Part model, mm, in its own coordinate system. A direction names the side the tool comes from. Give positions to 0.01 mm unless a question says otherwise; leave off trailing zeros. Write each loop counter-clockwise with the first axis right and the second up, starting at its lowest first coordinate (ties: lowest second). Pieces come first, ordered by that corner, then holes. Notation, with made-up numbers: (-23.75, 33) - (-10.75, 33) arc R9 cw to (-10.75, 48) - close; hole circle Ø2 at (47, 36). An arc over 180 degrees is marked (long way). Answer in a Markdown table with one row per item. Add a question column.
1. Band-saw the part on A-A on y = 8. State how many separate pieces and enclosed holes the cut face has, plus the area to 3 significant figures.
2. Pull direction Z, two halves, no side cores. Call faces 5 (the cylindrical face through (-5.08, -0.07, -25.92)), 6 (the cylindrical face through (-24.89, -0.07, 8.62)), 7 (the flat face through (24.3, 41, -39)): released by +Z, released by -Z, zero draft, split by the parting line, or undercut.
3. Band-saw the part on C-C on x = -4. Write the cut outline in (y, z).
4. Drop flat-ended pins along their axis: pin 1 Ø10 at (x, y) = (30.5, 23.5) entering from +Z; pin 2 Ø5 at (x, y) = (-39.5, -1) entering from +Z; pin 3 Ø1.5 at (x, z) = (-24, -2.5) entering from +Y. Give the stop position or say it passes through.
5. Probe line 1 along Z through (x, y) = (-23.75, 27.5); line 2 along Z through (x, y) = (0, 1); line 3 along Y through (x, z) = (-15, 32). List the from-to ranges inside material, lowest first.
6. Band-saw the part on B-B on z = 5. Write the cut outline in (x, y), plus the area to 3 significant figures.
7. Band-saw the part on D-D on x = -42. Write the cut outline in (y, z), plus the area to 3 significant figures.
8. Which spindle directions (+Z, -Z, +X, -X, +Y, -Y) get a long thin tool onto all of the face, cutting with end or side? Do faces 1 (the flat face through (12.522, 0.07, -36.689)), 2 (the cylindrical face through (24.89, -0.07, -8.62)), 3 (the cylindrical face through (-24.99, -0.07, -8.56)), 4 (the flat face through (-12.522, 0.07, 36.689)). Say none if no direction does.
```python
from build123d import *
from build123d.topology import SkipClean

# Parameters (mm, degrees)
SKETCH1_R                  = 25
SKETCH1_R_2                = 15
BOSS_EXTRUDE1_DEPTH        = 5
BOSS_EXTRUDE2_START        = -10
BOSS_EXTRUDE2_DEPTH        = 10
BOSS_EXTRUDE4_START        = 36
SKETCH8_R                  = 7.5
BOSS_EXTRUDE4_DEPTH        = 36
TAP_DRILL_FOR_10_32_TAP1_D = 4.0386
CIRPATTERN2_COUNT          = 6
FILLET1_R                  = 7.5


with BuildPart() as part:
    # Sketch1 → Boss-Extrude1 (new, symmetric)
    with BuildSketch(Plane(origin=(0, 0, 0), x_dir=(1, 0, 0), z_dir=(0, 1, 0))):
        with Locations(Location((0, 0, 0), (0, 0, 270))):
            Circle(SKETCH1_R)
        with Locations(Location((0, 0, 0), (0, 0, 270))):
            Circle(SKETCH1_R_2, mode=Mode.SUBTRACT)
    boss_extrude1 = extrude(amount=BOSS_EXTRUDE1_DEPTH, both=True)

    # Sketch2 → Boss-Extrude2 (add)
    with BuildSketch(Plane.XZ.offset(5).offset(BOSS_EXTRUDE2_START)):
        with BuildLine():
            ThreePointArc((55, 0), (52.803300859, 5.303300859), (47.5, 7.5))
            Line((47.5, 7.5), (23.848480035, 7.5))
            ThreePointArc((23.848480035, 7.5), (24.710443145, 3.793942482), (25, 0))
            ThreePointArc((25, 0), (24.710443145, -3.793942482), (23.848480035, -7.5))
            Line((23.848480035, -7.5), (47.5, -7.5))
            ThreePointArc((47.5, -7.5), (52.803300859, -5.303300859), (55, 0))
        make_face()
    boss_extrude2 = extrude(amount=BOSS_EXTRUDE2_DEPTH)

    # Sketch8 → Boss-Extrude4 (add)
    with SkipClean():  # the faces are left unmerged after this step: merging them gives an invalid solid
        with BuildSketch(Plane(origin=(0, 5, 0), x_dir=(1, 0, 0), z_dir=(0, 1, 0)).offset(BOSS_EXTRUDE4_START)):
            with Locations(Location((47.5, 0, 0), (0, 0, 270))):
                Circle(SKETCH8_R)
        boss_extrude4 = extrude(amount=-BOSS_EXTRUDE4_DEPTH)

    # Tap Drill for #10-32 Tap1 (through all)
    with Locations(Plane(origin=(0, -5, 0), x_dir=(-1, 0, 0), z_dir=(0, -1, 0))):
        with Locations((-47.5, 0)):
            tap_drill_for_10_32_tap1 = Hole(TAP_DRILL_FOR_10_32_TAP1_D / 2)

    # CirPattern2: Boss-Extrude1, Boss-Extrude2, Boss-Extrude4, Tap Drill for #10-32 Tap1 ×6 about axis
    cirpattern2_axis = Axis((0, 0, 0), (0, 1, 0))
    add([boss_extrude1.rotate(cirpattern2_axis, i * 360 / CIRPATTERN2_COUNT) for i in range(1, CIRPATTERN2_COUNT)])
    add([boss_extrude2.rotate(cirpattern2_axis, i * 360 / CIRPATTERN2_COUNT) for i in range(1, CIRPATTERN2_COUNT)])
    add([boss_extrude4.rotate(cirpattern2_axis, i * 360 / CIRPATTERN2_COUNT) for i in range(1, CIRPATTERN2_COUNT)])
    add([tap_drill_for_10_32_tap1.rotate(cirpattern2_axis, i * 360 / CIRPATTERN2_COUNT) for i in range(1, CIRPATTERN2_COUNT)], mode=Mode.SUBTRACT)

    # Fillet1
    fillet1_edges = [part.edges().sort_by_distance(p)[0] for p in [
        (23.848480035, 0, -7.5),
        (23.848480035, 0, 7.5),
        (18.419430546, 0, 16.903389552),
        (5.429049489, 0, 24.403389552),
        (-5.429049489, 0, 24.403389552),
        (-18.419430546, 0, 16.903389552),
        (-23.848480035, 0, 7.5),
        (-23.848480035, 0, -7.5),
        (-18.419430546, 0, -16.903389552),
        (-5.429049489, 0, -24.403389552),
        (5.429049489, 0, -24.403389552),
        (18.419430546, 0, -16.903389552),
    ]]
    fillet(fillet1_edges, radius=FILLET1_R)


solid = part.part
```
Values:
| question | item | result |
|---|---|---|
| 1 | separate pieces | 6 |
| 1 | enclosed holes | 6 |
| 1 | area | 983 mm² |
| 2 | face 5 | released by -Z |
| 2 | face 6 | undercut |
| 2 | face 7 | zero draft |
| 3 | outline | (-5, -25.42) - (5, -25.42) - (5, -14.46) - (-5, -14.46) - close; (-5, 14.46) - (5, 14.46) - (5, 25.42) - (-5, 25.42) - close |
| 4 | pin 1 | stops at z = 48.43 |
| 4 | pin 2 | stops at z = 7.5 |
| 4 | pin 3 | stops at y = 5 |
| 5 | line 1 | z = -48.64 to -43.16, -39.12 to -33.64, 33.64 to 39.12, 43.16 to 48.64 |
| 5 | line 2 | z = -25 to -15, 15 to 25 |
| 5 | line 3 | y = -5 to 5 |
| 6 | outline | (-53.09, -5) - (-14.14, -5) - (-14.14, 5) - (-41.91, 5) - (-41.91, 41) - (-53.09, 41) - close; (14.14, -5) - (53.09, -5) - (53.09, 41) - (41.91, 41) - (41.91, 5) - (14.14, 5) - close |
| 6 | area | 1,580 mm² |
| 7 | outline | (-5, -7.5) - (5, -7.5) - (5, -5.1) - (41, -5.1) - (41, 5.1) - (5, 5.1) - (5, 7.5) - (-5, 7.5) - close |
| 7 | area | 517 mm² |
| 8 | face 1 | -Z, +Y, -Y |
| 8 | face 2 | +X, +Y, -Y |
| 8 | face 3 | -X, +Y, -Y |
| 8 | face 4 | +Z, +Y, -Y |
